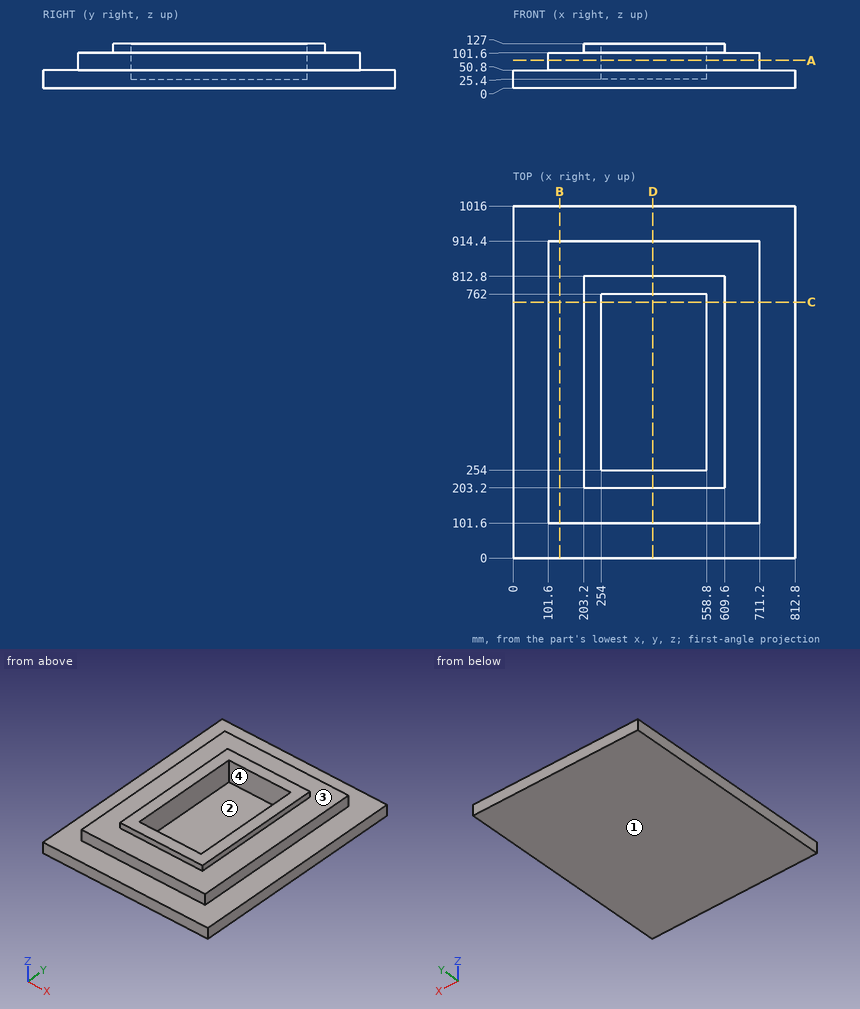
Can you work these out from the drawing? Everything is in mm from the part's minimum corner. A direction names the side the tool comes from. Coordinates: 2 decimals unless noted, no trailing zeros. Write each loop counter-clockwise with the first axis right and the second up, starting at its lowest first coordinate (ties: lowest second). Pieces come first, ordered by that corner, then holes. Notation, with made-up numbers: (7, -5) -> (33, -5) arc R24 ccw to (33, 16) -> close; hole circle Ø6 at (62, 79.5). An arc over 180 degrees is marked (long way). Write each question's results on one line, items separated by ' | '. Start each with the question number.
Q1. If I drill on probe 1 along Y at (x, z) = (456, 33); probe 2 along Y at (x, z) = (271, 61.5); probe 3 along X at (y, z) = (320.5, 107), over which ranges is the centre line in solid material (lowest first)?
Q2. Imagine slicing it at B-B (x = 134). Write out the boundary of the cut face in (y, z).
Q3. Imagine slicing it at D-D (x = 403). Write out the boundary of the cut face in (y, z).
Q4. We'd pull the mould along X, two halves only. Please class the marked faces 3 and 4: +X half, -X half, draft (parallel to the pull), parting line (faces both ways), or undercut.
Q5. On a 3-axis mill with a long thin cutter (end or side, diameter ignored), from which of +Z, -Z, +X, -X, +Y, -Y can I reach the whole of each face in a straight line? I mean the marked faces 1 and 2. Say none if no direction works.
Q6. Imagine slicing it at A-A (z = 80). Write out the boundary of the cut face in (x, y).
Q7. Imagine slicing it at C-C (y = 738.5). Write out the boundary of the cut face in (x, z).
Q8. I'm going to push flat-ended pins straight in: pin 1 (8 mm diameter, centred on x = 609.5, z = 69.5, fed in from -Y); pin 2 (7.5 mm diameter, centred on x = 387, z = 120.5, fed in from -Y); pin 3 (1 mm diameter, centred on y = 878, z = 103, fed in from -X) (3 decimals); pin 4 (8 mm diameter, centred on y = 509.5, z = 96.5, fed in from +X). Where does each tip first touch, or does it pass through?
Taken from the geometry:
1) probe 1: y = 0 to 254, 762 to 1016 | probe 2: y = 101.6 to 254, 762 to 914.4 | probe 3: x = 203.2 to 254, 558.8 to 609.6
2) outline: (0, 0) -> (1016, 0) -> (1016, 50.8) -> (914.4, 50.8) -> (914.4, 101.6) -> (101.6, 101.6) -> (101.6, 50.8) -> (0, 50.8) -> close
3) outline: (0, 0) -> (1016, 0) -> (1016, 50.8) -> (914.4, 50.8) -> (914.4, 101.6) -> (812.8, 101.6) -> (812.8, 127) -> (762, 127) -> (762, 25.4) -> (254, 25.4) -> (254, 127) -> (203.2, 127) -> (203.2, 101.6) -> (101.6, 101.6) -> (101.6, 50.8) -> (0, 50.8) -> close
4) face 3: draft | face 4: undercut
5) face 1: -Z, +X, -X, +Y, -Y | face 2: +Z
6) outline: (101.6, 101.6) -> (711.2, 101.6) -> (711.2, 914.4) -> (101.6, 914.4) -> close; hole (254, 254) -> (558.8, 254) -> (558.8, 762) -> (254, 762) -> close
7) outline: (0, 0) -> (812.8, 0) -> (812.8, 50.8) -> (711.2, 50.8) -> (711.2, 101.6) -> (609.6, 101.6) -> (609.6, 127) -> (558.8, 127) -> (558.8, 25.4) -> (254, 25.4) -> (254, 127) -> (203.2, 127) -> (203.2, 101.6) -> (101.6, 101.6) -> (101.6, 50.8) -> (0, 50.8) -> close
8) pin 1: stops at y = 101.6 | pin 2: stops at y = 203.2 | pin 3: passes through | pin 4: stops at x = 711.2
